```python
from build123d import *

# Parameters (mm, degrees)
F0_W      = 12.7
F0_H      = 6.35
F1_DEPTH  = 6.35
F2_W      = 12.7
F2_H      = 6.35
F3_DEPTH  = 3.175
F4_W      = 6.35
F4_H      = 6.35
F5_DEPTH  = 12.7
F6_R      = 9.525
F6_W      = 15.875
F6_H      = 6.35
F7_DEPTH  = 3.175
F8_R      = 9.525
F9_DEPTH  = 3.175
F10_R     = 9.525
F11_DEPTH = 3.175
F12_R     = 9.525
F13_DEPTH = 3.175


# Not quite as in the source:
# - a feature names something its author has since deleted; it is built from what else it names


with BuildPart() as f1:
    # F0 (on Front) → F1 (new body)
    with BuildSketch(Plane.XZ):
        with Locations((6.35, 3.175)):
            Rectangle(F0_W, F0_H)
    extrude(amount=F1_DEPTH)

    # F2 (on face) → F3 (join)
    with BuildSketch(Plane.XZ.offset(6.35)):
        with Locations((-6.35, 3.175)):
            Rectangle(F2_W, F2_H)
        with Locations((6.35, 3.175)):
            Rectangle(F2_W, F2_H)
        with Locations((19.05, 3.175)):
            Rectangle(F2_W, F2_H)
    extrude(amount=F3_DEPTH)

    # F4 (on face) → F5 (join)
    with BuildSketch(Plane.XZ.offset(9.525)):
        with Locations((-9.525, 3.175)):
            Rectangle(F4_W, F4_H)
        with Locations((22.225, 3.175)):
            Rectangle(F4_W, F4_H)
    extrude(amount=F5_DEPTH)

    # F6 (on face) → F7 (join)
    with BuildSketch(Plane.YZ.offset(25.4)):
        with Locations((-14.2875, 3.175)):
            Circle(F6_R)
        with Locations((-14.2875, 3.175)):
            Rectangle(F6_W, F6_H, mode=Mode.SUBTRACT)
        with Locations((-14.2875, 3.175)):
            Rectangle(F6_W, F6_H)
    extrude(amount=F7_DEPTH)

    # F8 (on face) → F9 (join)
    with BuildSketch(Plane(origin=(-12.7, 0, 0), x_dir=(0, -1, 0), z_dir=(-1, 0, 0))):
        with Locations((14.2875, 3.175)):
            Circle(F8_R)
    extrude(amount=F9_DEPTH)

    # F10 (on face) → F11 (join)
    with BuildSketch(Plane(origin=(19.05, 0, 0), x_dir=(0, -1, 0), z_dir=(-1, 0, 0))):
        with Locations((15.875, 3.175)):
            Circle(F10_R)
    extrude(amount=F11_DEPTH)

    # F12 (on face) → F13 (join)
    with BuildSketch(Plane.YZ.offset(-6.35)):
        with Locations((-15.875, 3.175)):
            Circle(F12_R)
    extrude(amount=F13_DEPTH)


solid = f1.part
```
Design review of the part built by this model. Coordinates are the model's own, in mm. A direction names the side the tool comes from. Coordinates: 2 decimals unless noted, no trailing zeros. Loops run counter-clockwise (first coordinate to the right, second up) from the corner with the lowest first, then second, coordinate; pieces in that order, holes last. Notation, with made-up numbers: (37.5, 43) - (74.5, 43) arc R32 ccw to (74.5, 72) - close; hole circle Ø2 at (45, -13.75). An arc over 180 degrees is marked (long way). Use CSV: the item, a comma, the result in double quotes. Start each with the question number.
1) For pin 1 Ø5 at (x, z) = (9.5, -0.5) entering from +Y; pin 2 Ø5 at (x, z) = (13.5, 7) entering from -Y; pin 3 Ø2 at (x, y) = (-8, -9) entering from +Z; pin 4 Ø1.9 at (x, z) = (18.5, 2) entering from +Y, all flat-tipped, find the tip position at first contact; note any pin that passes through.
2) The part is to be moulded in two halves that separate along X. For faces 4 (the cylindrical face through (26.97, -21.31, 9.61)), 5 (the flat face through (6, -9.525, 3)), say which applies: +X half, -X half, draft (parallel to the pull), parting line (faces both ways), or undercut.
3) Consider section A-A on z = 10.5. Write out the cut boundary in (x, y) (3 decimals), then the cut area to 3 significant figures.
4) Tool access review of faces 1 (the cylindrical face through (17.485, -25.393, 2.801)), 2 (the flat face through (12.7, -3, 3)), 3 (the flat face through (-10, -22.225, 3)): name each direction out of +Z, -Z, +X, -X, +Y, -Y from which nothing blocks a thin tool from reaching the whole face with its end or side.
5) Consider section D-D on x = 24.5. Write out the cut boundary in (y, z) (3 decimals).
6) Consider section B-B on y = -16.5. Write out the cut boundary in (x, z) (3 decimals).
7) Wall thickness on L1, parallel to X at y = -13.75, z = -5 (3 decimals); L2, parallel to X at y = -14.75, z = 4.25 (3 decimals); L3, parallel to X at y = -9.5, z = -4.25 (3 decimals): over which ranges is each line inside the solid? List them lowest first. Write a range as from..to.
8) Consider section C-C on z = 1.5. Write out the cut boundary in (x, y) (3 decimals).
Geometry says:
1,pin 1,"y = 0"
1,pin 2,"y = -24.9"
1,pin 3,"z = 6.35"
1,pin 4,"y = -6.35"
2,face 4,"draft"
2,face 5,"undercut"
3,outline,"(-15.875, -20.376) - (-12.7, -20.376) - (-12.7, -8.199) - (-15.875, -8.199) - close; (-6.35, -21.964) - (-3.175, -21.964) - (-3.175, -9.786) - (-6.35, -9.786) - close; (15.875, -21.964) - (19.05, -21.964) - (19.05, -9.786) - (15.875, -9.786) - close; (25.4, -20.376) - (28.575, -20.376) - (28.575, -8.199) - (25.4, -8.199) - close"
3,area,"155 mm^2"
4,face 1,"none"
4,face 2,"+Z, -Z, +Y"
4,face 3,"+Z, -Z, -Y"
5,outline,"(-22.225, 0) - (-6.35, 0) - (-6.35, 6.35) - (-22.225, 6.35) - close"
6,outline,"(-15.875, -6.089) - (-12.7, -6.089) - (-12.7, 0) - (-6.35, 0) - (-6.35, -6.329) - (-3.175, -6.329) - (-3.175, 12.679) - (-6.35, 12.679) - (-6.35, 6.35) - (-12.7, 6.35) - (-12.7, 12.439) - (-15.875, 12.439) - close; (15.875, -6.329) - (19.05, -6.329) - (19.05, 0) - (25.4, 0) - (25.4, -6.089) - (28.575, -6.089) - (28.575, 12.439) - (25.4, 12.439) - (25.4, 6.35) - (19.05, 6.35) - (19.05, 12.679) - (15.875, 12.679) - close"
7,L1,"-15.875..-12.7, -6.35..-3.175, 15.875..19.05, 25.4..28.575"
7,L2,"-15.875..-3.175, 15.875..28.575"
7,L3,"-15.875..-12.7, 25.4..28.575"
8,outline,"(-15.875, -23.664) - (-12.7, -23.664) - (-12.7, -22.225) - (-6.35, -22.225) - (-6.35, -25.252) - (-3.175, -25.252) - (-3.175, -9.525) - (15.875, -9.525) - (15.875, -25.252) - (19.05, -25.252) - (19.05, -22.225) - (25.4, -22.225) - (25.4, -23.664) - (28.575, -23.664) - (28.575, -4.911) - (25.4, -4.911) - (25.4, -6.35) - (12.7, -6.35) - (12.7, 0) - (0, 0) - (0, -6.35) - (-12.7, -6.35) - (-12.7, -4.911) - (-15.875, -4.911) - close"
